CAD build for the part. Positions are in the model's coordinates, mm. Give positions to 0.01 mm unless a question says otherwise; leave off trailing zeros. Loops run counter-clockwise (first coordinate to the right, second up) from the corner with the lowest first, then second, coordinate; pieces in that order, holes last. Notation, with made-up numbers: (9.25, -30) - (31.25, -30) arc R19 ccw to (31.25, -4) - close; hole circle Ø2 at (77.5, 67.5). An arc over 180 degrees is marked (long way). Return JSON: item names as keys, results as strings.
Autodesk Inventor part; units mm, degrees
ref_plane "Plano inicial" through (0, 0, 0) normal (0, 0, 1) x (1, 0, 0)
ref_plane "Plano final" through (0, 0, 630) normal (0, 0, 1) x (1, 0, 0)
ref_plane "YZ Plane" through (0, 0, 0) normal (1, 0, 0) x (0, 1, 0)
ref_plane "Plano inicial" through (0, 0, 0) normal (0, 0, 1) x (1, 0, 0)
ref_plane "Plano final" through (0, 0, 630) normal (0, 0, 1) x (1, 0, 0)
sketch "Boceto" plane through (0, 0, 0) normal (0, 0, 1) x (1, 0, 0)
  line L0 (-14.2, 20) -> (14.2, 20)
  line L1 (20, 14.2) -> (20, -14.2)
  line L2 (14.2, -20) -> (-14.2, -20)
  line L3 (-20, -14.2) -> (-20, 14.2)
  arc A0 (-14.2, 20) -> (-20, 14.2) centre (-14.2, 14.2) ccw
  arc A1 (20, 14.2) -> (14.2, 20) centre (14.2, 14.2) ccw
  arc A2 (14.2, -20) -> (20, -14.2) centre (14.2, -14.2) ccw
  arc A3 (-20, -14.2) -> (-14.2, -20) centre (-14.2, -14.2) ccw
  line L4 (-29.6817, 0) -> (29.6817, 0) construction
  line L5 (0, -29.6817) -> (0, 29.6817) construction
  arc A4 (-14.2, 17.1) -> (-17.1, 14.2) centre (-14.2, 14.2) ccw
  line L6 (-14.2, 17.1) -> (14.2, 17.1)
  arc A5 (17.1, 14.2) -> (14.2, 17.1) centre (14.2, 14.2) ccw
  line L7 (17.1, 14.2) -> (17.1, -14.2)
  arc A6 (14.2, -17.1) -> (17.1, -14.2) centre (14.2, -14.2) ccw
  line L8 (14.2, -17.1) -> (-14.2, -17.1)
  arc A7 (-17.1, -14.2) -> (-14.2, -17.1) centre (-14.2, -14.2) ccw
  line L9 (-17.1, -14.2) -> (-17.1, 14.2)
  point P0 (-20, 20)
  point P1 (20, -20)
  point P2 (20, 20)
  dimension "b" = 40
  dimension "msp_r" = 5.8
  dimension "d8" = 20
  dimension "d9" = 20
  dimension "d10" = 2.9
extrude "Cuerpo" add sketch "Boceto" along normal up to surface (630 mm away) from surface at 0
sketch "Sketch2" plane through (0, 0, 0) normal (0, 0, 1) x (1, 0, 0)
  line L0 (0, 0) -> (10, 0)
ref_plane "Work Plane3" through (0, 0, 0) normal (0, -1, 0) x (1, 0, 0)
sketch "Sketch3" plane through (0, 0, 0) normal (0, -1, 0) x (1, 0, 0)
  line L0 (-2, 0) -> (12, 0)
  line L1 (-2, 630) -> (12, 630)
  dimension "d14" = 630
equation "\"msp_r\" = 2 * ParT"
equation "\"d8\" = d9"
equation "\"d9\" = 0.5 * b"
equation "\"d10\" = ParT"
equation "\"G_OFFSET_START\" = 0"
equation "\"G_OFFSET_END\" = 0"
equation "\"G_L\" = d14"
properties part number "DIN 59 410 - 40x40x2.9-630" material "Acero, suave"
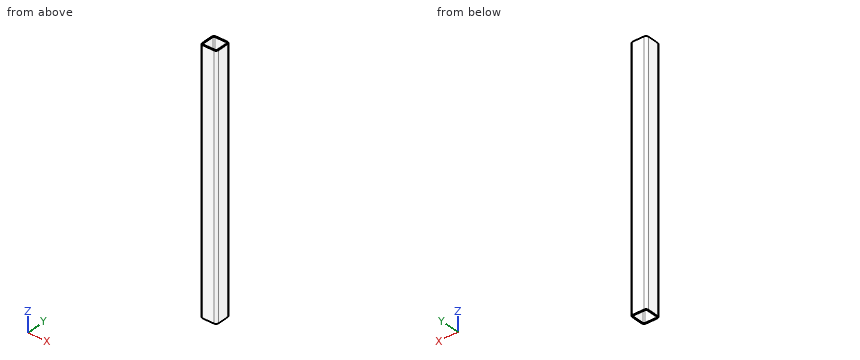
1. Cut at C-C, the plane z = 106.5. Write the cut outline in (x, y), plus the area to 3 significant figures.
Values follow:
{"outline": "(-20, -14.2) arc R5.8 ccw to (-14.2, -20) - (14.2, -20) arc R5.8 ccw to (20, -14.2) - (20, 14.2) arc R5.8 ccw to (14.2, 20) - (-14.2, 20) arc R5.8 ccw to (-20, 14.2) - close; hole (-17.1, -14.2) arc R2.9 ccw to (-14.2, -17.1) - (14.2, -17.1) arc R2.9 ccw to (17.1, -14.2) - (17.1, 14.2) arc R2.9 ccw to (14.2, 17.1) - (-14.2, 17.1) arc R2.9 ccw to (-17.1, 14.2) - close", "area": "409 mm²"}
2. Cut at A-A, the plane y = 9. Write the cut outline in (x, z), plus the area to 3 significant figures.
Values follow:
{"outline": "(-20, 0) - (-17.1, 0) - (-17.1, 630) - (-20, 630) - close; (17.1, 0) - (20, 0) - (20, 630) - (17.1, 630) - close", "area": "3,650 mm²"}
3. Drill centre lines: probe 1 along X at (y, z) = (14, 308); probe 2 along X at (y, z) = (15.5, 160). Where is each one in solid material? Low to high.
Values follow:
{"probe 1": "x = -20 to -17.1, 17.1 to 20", "probe 2": "x = -19.85 to -16.79, 16.79 to 19.85"}
